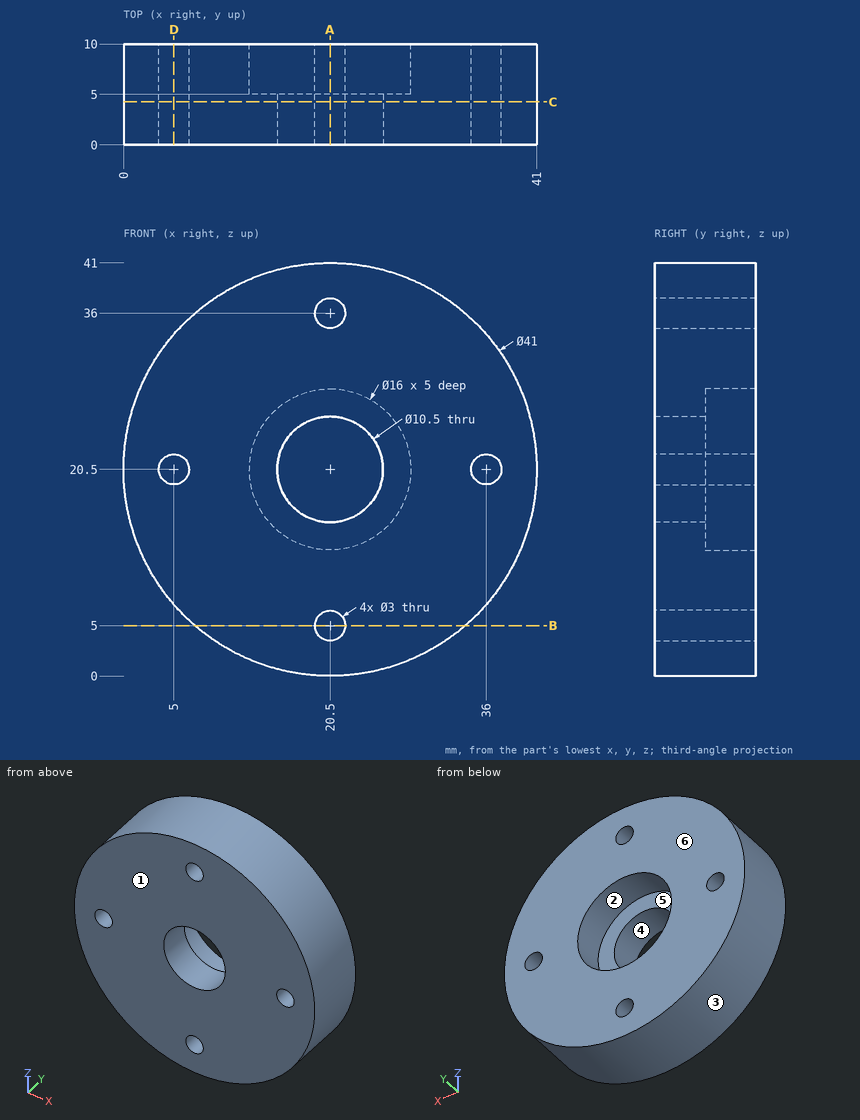
The drawing under review shows one solid part. Ordinate dimensions are in mm from its lowest x, y, z. A direction names the side the tool comes from. Coordinates: 2 decimals unless noted, no trailing zeros. Write each loop counter-clockwise with the first axis right and the second up, starting at its lowest first coordinate (ties: lowest second). Pieces come first, ordered by that corner, then holes.
1) Machinability: for the marked faces 5 and 6, which of the approach directions +Z, -Z, +X, -X, +Y, -Y give a long, thin tool a straight path to every point of the face, cutting with its end or side? Answer none if there is none.
2) Add section C-C (y = 4.25). Write out the cut boundary in (x, z), plus the area to 3 significant figures.
3) Add section A-A (x = 20.5). Write out the cut boundary in (y, z).
4) Add section B-B (z = 5). Write out the cut boundary in (x, y).
5) To check wall thickness, follow L1, parallel to Y at x = 22.5, z = 27; L2, parallel to Z at x = 24, y = 1.75; L3, parallel to X at y = 2.5, z = 5. State the ranges of each line that lie inside material, in increasing order.
6) Add section D-D (x = 5). Write out the cut boundary in (y, z), plus the area to 3 significant figures.
7) Mouldability with a two-part tool opening along X and no side actions: class the marked faces 1, 2, 3 and 4 as +X half, -X half, draft (parallel to the pull), parting line (faces both ways), or undercut.
8) Insertion check: pin 1 (4 mm diameter, centred on x = 21, y = 4, fed in from -Z); pin 2 (4 mm diameter, centred on y = 1.5, z = 22, fed in from -X); pin 3 (3 mm diameter, centred on y = 3, z = 16.5, fed in from -X); pin 4 (8.5 mm diameter, centred on x = 20.5, z = 20.5, fed in from +Y). Each pin has a flat end and moves straight along its axis. Give the tip position at first contact, or say it passes through.
Check result:
1. face 5: +Y
1. face 6: +Z, -Z, +X, -X, +Y
2. outline: circle Ø41 at (20.5, 20.5); hole circle Ø3 at (5, 20.5); hole circle Ø10.5 at (20.5, 20.5); hole circle Ø3 at (20.5, 5); hole circle Ø3 at (20.5, 36); hole circle Ø3 at (36, 20.5)
2. area: 1,210 mm2
3. outline: (0, 0) - (10, 0) - (10, 3.5) - (0, 3.5) - close; (0, 6.5) - (10, 6.5) - (10, 12.5) - (5, 12.5) - (5, 15.25) - (0, 15.25) - close; (0, 25.75) - (5, 25.75) - (5, 28.5) - (10, 28.5) - (10, 34.5) - (0, 34.5) - close; (0, 37.5) - (10, 37.5) - (10, 41) - (0, 41) - close
4. outline: (7.08, 0) - (19, 0) - (19, 10) - (7.08, 10) - close; (22, 0) - (33.92, 0) - (33.92, 10) - (22, 10) - close
5. L1: y = 0 to 5
5. L2: z = 0.3 to 16.59, 24.41 to 40.7
5. L3: x = 7.08 to 19, 22 to 33.92
6. outline: (0, 7.08) - (10, 7.08) - (10, 19) - (0, 19) - close; (0, 22) - (10, 22) - (10, 33.92) - (0, 33.92) - close
6. area: 238 mm2
7. face 1: draft
7. face 2: undercut
7. face 3: parting line
7. face 4: undercut
8. pin 1: stops at z = 0
8. pin 2: stops at x = 0
8. pin 3: stops at x = 0.15
8. pin 4: passes through
